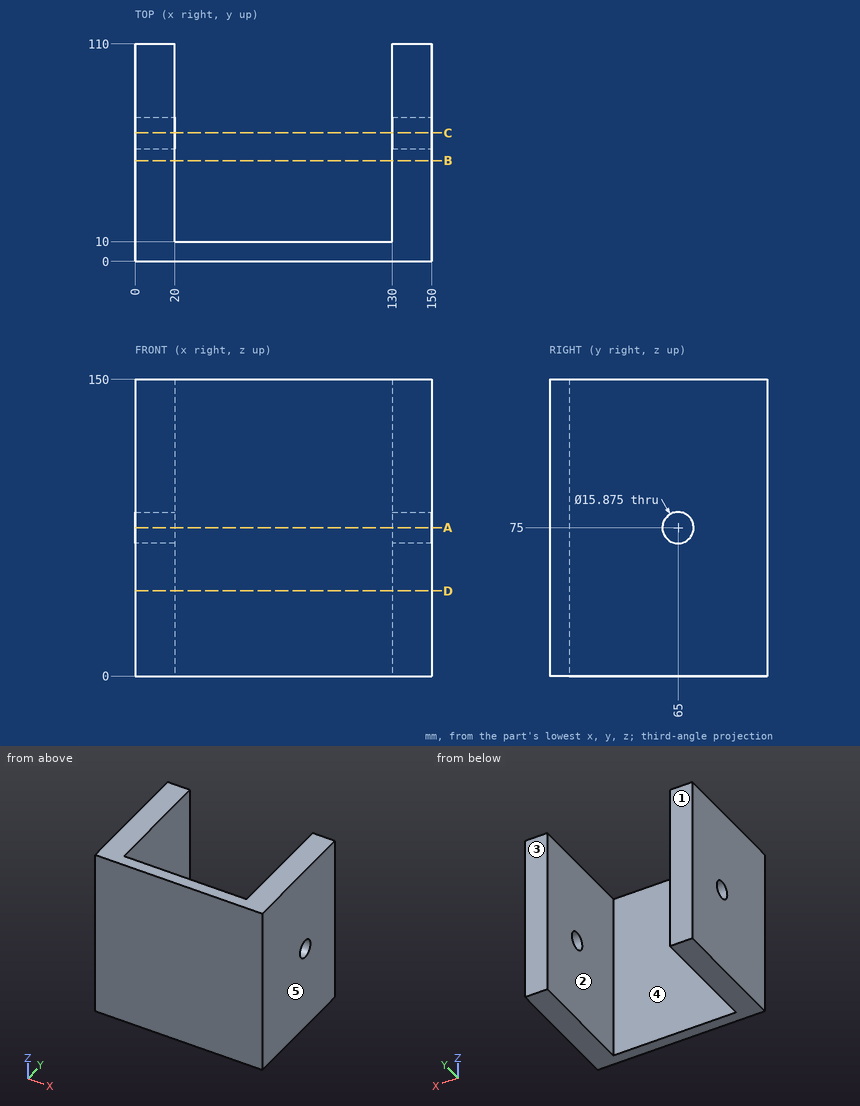
Print and shaded views of the part. All mm, measured from the part's lowest x, y and z. A direction names the side the tool comes from. Coordinates: 2 decimals unless noted, no trailing zeros. Loops run counter-clockwise (first coordinate to the right, second up) from the corner with the lowest first, then second, coordinate; pieces in that order, holes last. Notation, with made-up numbers: M -35.5,28 L 11.5,28 A26 cw 11.5,47 Z; hole C 77.25,32.25 d5. An arc over 180 degrees is marked long. Use a Markdown table: item, result. Add a question column.
Q1. Cut at C-C (y = 65). Write the cut outline in (x, z), and give its area (4 significant figures).
Q2. Pin check, flat tip, straight feed: P1, Ø8, axis at x = 33, z = 40.5, coming from the +Y side. Stop position of the tip, or through.
Q3. Cut at A-A (z = 75). Write the cut outline in (x, y), and give its area (4 significant figures).
Q4. Which spindle directions (+Z, -Z, +X, -X, +Y, -Y) get a long thin tool onto all of the face, cutting with end or side? Do the marked faces 1 and 2. Say none if no direction does.
Q5. Cut at D-D (z = 43). Write the cut outline in (x, y).
Q6. Cut at B-B (y = 51). Write the cut outline in (x, z).
Q7. Mould opens along X. For the marked faces 3, 4 and 5 say: +X half, -X half, draft (parallel to the pull), parting line (faces both ways), or undercut.
Q8. Probe L1, parallel to X at y = 45, z = 131; L2, parallel to Y at x = 136, z = 75; L3, parallel to Z at x = 14, y = 59. List the from-to ranges inside material, lowest first.
Worked out:
| question | item | result |
|---|---|---|
| 1 | outline | M 0,0 L 20,0 L 20,67.06 L 0,67.06 Z; M 0,82.94 L 20,82.94 L 20,150 L 0,150 Z; M 130,0 L 150,0 L 150,67.06 L 130,67.06 Z; M 130,82.94 L 150,82.94 L 150,150 L 130,150 Z |
| 1 | area | 5,365 mm2 |
| 2 | P1 | stops at y = 10 |
| 3 | outline | M 0,0 L 150,0 L 150,57.06 L 130,57.06 L 130,10 L 20,10 L 20,57.06 L 0,57.06 Z; M 0,72.94 L 20,72.94 L 20,110 L 0,110 Z; M 130,72.94 L 150,72.94 L 150,110 L 130,110 Z |
| 3 | area | 4,865 mm2 |
| 4 | face 1 | +Z, -Z, +X, -X, +Y |
| 4 | face 2 | +Z, -Z, +Y |
| 5 | outline | M 0,0 L 150,0 L 150,110 L 130,110 L 130,10 L 20,10 L 20,110 L 0,110 Z |
| 6 | outline | M 0,0 L 20,0 L 20,150 L 0,150 Z; M 130,0 L 150,0 L 150,150 L 130,150 Z |
| 7 | face 3 | draft |
| 7 | face 4 | undercut |
| 7 | face 5 | +X half |
| 8 | L1 | x = 0 to 20, 130 to 150 |
| 8 | L2 | y = 0 to 57.06, 72.94 to 110 |
| 8 | L3 | z = 0 to 69.8, 80.2 to 150 |
